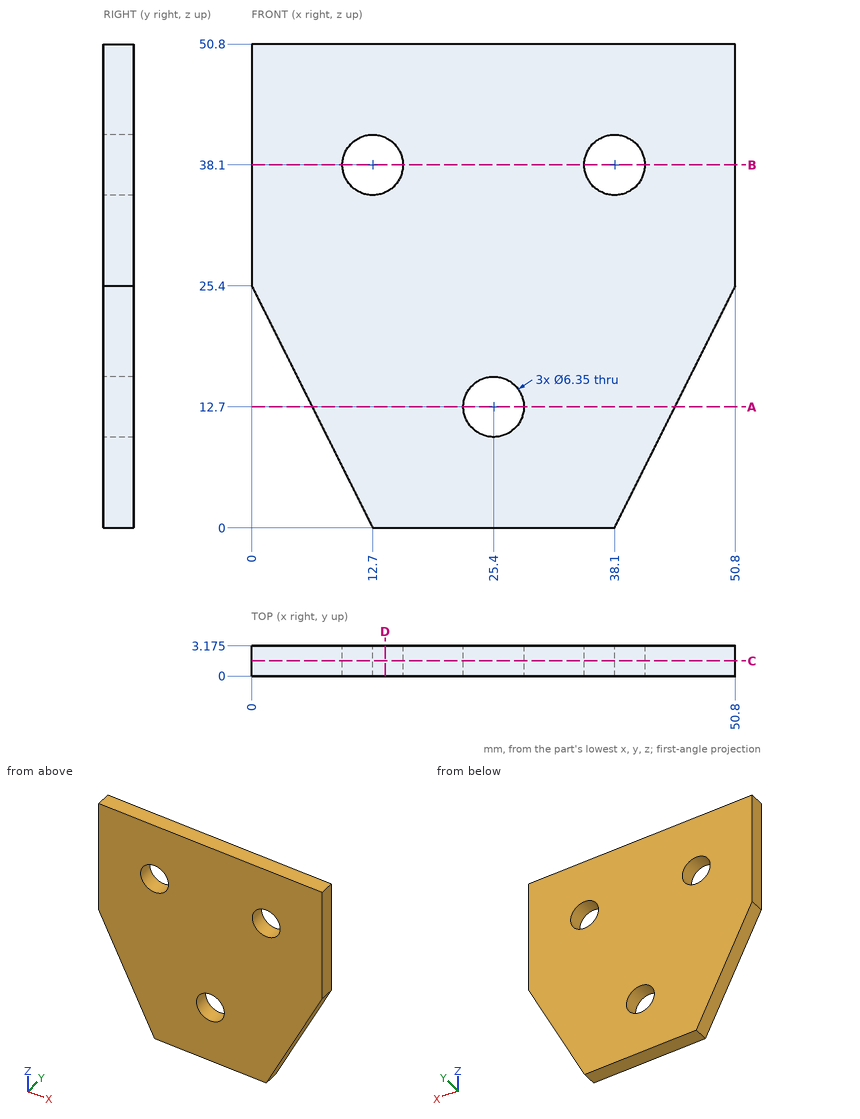
Input: dimensioned drawing with shaded views. Units: mm. Origin: part minimum x, y, z. Give positions to 0.01 mm unless a question says otherwise; leave off trailing zeros. Write each loop counter-clockwise with the first axis right and the second up, starting at its lowest first coordinate (ties: lowest second). Pieces come first, ordered by that corner, then holes. Notation, with made-up numbers: (-36, 74) -> (17, 74) arc R30 cw to (17, 106) -> close; hole circle Ø3 at (26, 47). An arc over 180 degrees is marked (long way). Return JSON: item names as keys, results as strings. Group by question number.
1. Section D-D, the plane x = 14. Output: boundary loops of the cut face in (y, z) (3 decimals).
2. Section A-A, the plane z = 12.7. Output: boundary loops of the cut face in (x, y) (3 decimals).
3. Section C-C, the plane y = 1.6. Output: boundary loops of the cut face in (x, z) (3 decimals), then the cut area to 3 significant figures.
4. Section B-B, the plane z = 38.1. Output: boundary loops of the cut face in (x, y) (3 decimals), then the cut area to 3 significant figures.
5. Material intervals for line 1 (Z direction, x = 25.4, y = 1.05) (3 decimals); line 2 (Z direction, x = 39.5, y = 2.8); line 3 (X direction, y = 0.35, z = 14.5), sorted ascending. Write a range as from..to.
Determined:
{
 "1": {"outline": "(0, 0) -> (3.175, 0) -> (3.175, 35.203) -> (0, 35.203) -> close; (0, 40.997) -> (3.175, 40.997) -> (3.175, 50.8) -> (0, 50.8) -> close"},
 "2": {"outline": "(6.35, 0) -> (22.225, 0) -> (22.225, 3.175) -> (6.35, 3.175) -> close; (28.575, 0) -> (44.45, 0) -> (44.45, 3.175) -> (28.575, 3.175) -> close"},
 "3": {"outline": "(0, 25.4) -> (12.7, 0) -> (38.1, 0) -> (50.8, 25.4) -> (50.8, 50.8) -> (0, 50.8) -> close; hole circle Ø6.35 at (12.7, 38.1); hole circle Ø6.35 at (25.4, 12.7); hole circle Ø6.35 at (38.1, 38.1)", "area": "2,160 mm2"},
 "4": {"outline": "(0, 0) -> (9.525, 0) -> (9.525, 3.175) -> (0, 3.175) -> close; (15.875, 0) -> (34.925, 0) -> (34.925, 3.175) -> (15.875, 3.175) -> close; (41.275, 0) -> (50.8, 0) -> (50.8, 3.175) -> (41.275, 3.175) -> close", "area": "121 mm2"},
 "5": {"line 1": "z = 0..9.525, 15.875..50.8", "line 2": "z = 2.8..35.25, 40.95..50.8", "line 3": "x = 5.45..22.78, 28.02..45.35"}
}
